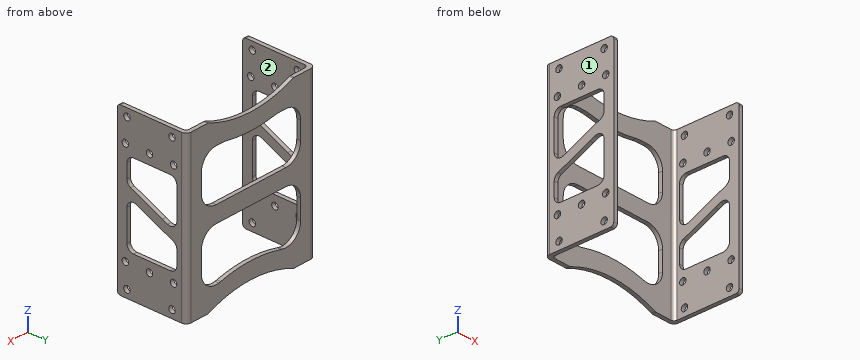
```python
from build123d import *

# Parameters (mm, degrees)
SKETCH_1_W                = 43.5
SKETCH_1_H                = 50
EXTRUDE_1_DEPTH           = 21.5
SKETCH_2_W                = 41.1
SKETCH_2_H                = 22.668209098
CUT_EXTRUDE_1_DEPTH       = 59.078072454
CUT_EXTRUDE_2_DEPTH       = 44.546670366
CUT_EXTRUDE_3_DEPTH       = 44.546670366
HOLE_WIZARD_2_0_2_1_D     = 2
HOLE_WIZARD_2_0_2_1_DEPTH = 1.2
HOLE_WIZARD_2_0_2_2_D     = 2
FILLET_1_R                = 1
FILLET_2_R                = 1.5
FILLET_3_R                = 1
CUT_EXTRUDE_5_DEPTH       = 10
FILLET_4_R                = 10
FILLET_5_R                = 5
CUT_EXTRUDE_6_DEPTH       = 58.037268572
FILLET_6_R                = 2
FILLET_7_R                = 2


with BuildPart() as part:
    # 草图1 → 凸台-拉伸1 (new body)
    with BuildSketch(Plane.XZ.offset(20)):
        with Locations((0, -6)):
            Rectangle(SKETCH_1_W, SKETCH_1_H)
    extrude(amount=-EXTRUDE_1_DEPTH)

    # 草图2 → 切除-拉伸1 (cut, through all)
    with BuildSketch(Plane.XY.offset(19)):
        with Locations((0, -11.034104549)):
            Rectangle(SKETCH_2_W, SKETCH_2_H)
    extrude(amount=-CUT_EXTRUDE_1_DEPTH, mode=Mode.SUBTRACT)

    # 草图3 → 切除-拉伸2 (cut, through all)
    with BuildSketch(Plane(origin=(0, 1.5, 0), x_dir=(-1, 0, 0), z_dir=(0, 1, 0))):
        with BuildLine():
            Line((14.38749457, 19), (-14.38749457, 19))
            ThreePointArc((-14.38749457, 19), (0, 16), (14.38749457, 19))
        make_face()
    extrude(amount=-CUT_EXTRUDE_2_DEPTH, mode=Mode.SUBTRACT)

    # 草图4 → 切除-拉伸3 (cut, through all)
    with BuildSketch(Plane(origin=(0, 1.5, 0), x_dir=(-1, 0, 0), z_dir=(0, 1, 0))):
        with BuildLine():
            Line((-14.38749457, -31), (14.38749457, -31))
            ThreePointArc((14.38749457, -31), (0, -28), (-14.38749457, -31))
        make_face()
    extrude(amount=-CUT_EXTRUDE_3_DEPTH, mode=Mode.SUBTRACT)

    # Ø2.0 (2) 直径孔1
    with Locations(Plane.ZY.offset(-20.55)):
        with Locations((16.6, -3), (16.6, -17), (9.5, -17.5), (9.6, -10), (9.5, -2.5), (-21.5, -2.5), (-28.6, -3), (-28.6, -17), (-21.5, -17.5), (-21.6, -10)):
            Hole(HOLE_WIZARD_2_0_2_1_D / 2, depth=HOLE_WIZARD_2_0_2_1_DEPTH)

    # Ø2.0 (2) 直径孔2 (through all)
    with Locations(Plane(origin=(-20.55, 0, 0), x_dir=(0, 0, -1), z_dir=(1, 0, 0))):
        with Locations((-16.6, -3), (-16.6, -17), (-9.5, -17.5), (-9.6, -10), (-9.5, -2.5), (21.5, -2.5), (28.6, -3), (28.6, -17), (21.5, -17.5), (21.6, -10)):
            Hole(HOLE_WIZARD_2_0_2_2_D / 2)

    # 圆角1
    fillet_1_edges = [part.edges().sort_by_distance(p)[0] for p in [
        (-21.15, -20, 19),
        (21.15, -20, -31),
        (-14.38749457, 0.9, 19),
        (14.38749457, 0.9, 19),
        (-21.15, -20, -31),
        (14.38749457, 0.9, -31),
        (-14.38749457, 0.9, -31),
        (21.15, -20, 19),
    ]]
    fillet(fillet_1_edges, radius=FILLET_1_R)

    # 圆角2
    fillet_2_edges = [part.edges().sort_by_distance(p)[0] for p in [
        (-21.75, 1.5, -6),
        (21.75, 1.5, -6),
    ]]
    fillet(fillet_2_edges, radius=FILLET_2_R)

    # 圆角3
    fillet_3_edges = [part.edges().sort_by_distance(p)[0] for p in [
        (-20.55, 0.3, -6),
        (20.55, 0.3, -6),
    ]]
    fillet(fillet_3_edges, radius=FILLET_3_R)

    # 草图14 → 切除-拉伸5 (cut)
    with BuildSketch(Plane(origin=(0, 1.5, 0), x_dir=(1, 0, 0), z_dir=(0, 1, 0))):
        with BuildLine():
            Line((-11.33348239, 24.597561282), (-16.75, 24.597561282))
            Line((-16.75, 24.597561282), (-16.75, 8.5))
            Line((-16.75, 8.5), (16.75, 8.5))
            Line((16.75, 8.5), (16.75, 24.597561282))
            Line((16.75, 24.597561282), (11.33348239, 24.597561282))
            ThreePointArc((11.33348239, 24.597561282), (0, 23), (-11.33348239, 24.597561282))
        make_face()
        with BuildLine():
            Line((16.75, 3.5), (-16.75, 3.5))
            Line((-16.75, 3.5), (-16.75, -11.921871339))
            Line((-16.75, -11.921871339), (-8.645438281, -11.921871339))
            ThreePointArc((-8.645438281, -11.921871339), (0, -11), (8.645438281, -11.921871339))
            Line((8.645438281, -11.921871339), (16.75, -11.921871339))
            Line((16.75, -11.921871339), (16.75, 3.5))
        make_face()
    extrude(amount=-CUT_EXTRUDE_5_DEPTH, mode=Mode.SUBTRACT)

    # 圆角4
    fillet_4_edges = [part.edges().sort_by_distance(p)[0] for p in [
        (-11.33348239, 0.9, -24.597561282),
        (11.33348239, 0.9, -24.597561282),
        (8.645438281, 0.9, 11.921871339),
        (-8.645438281, 0.9, 11.921871339),
    ]]
    fillet(fillet_4_edges, radius=FILLET_4_R)

    # 圆角5
    fillet_5_edges = [part.edges().sort_by_distance(p)[0] for p in [
        (-16.75, 0.9, 11.921871339),
        (-16.75, 0.9, -3.5),
        (16.75, 0.9, 11.921871339),
        (16.75, 0.9, -3.5),
        (16.75, 0.9, -8.5),
        (16.75, 0.9, -24.597561282),
        (-16.75, 0.9, -8.5),
        (-16.75, 0.9, -24.597561282),
    ]]
    fillet(fillet_5_edges, radius=FILLET_5_R)

    # 草图15 → 切除-拉伸6 (cut, through all)
    with BuildSketch(Plane.ZY.offset(21.75)):
        Polygon((-11, -1.5), (-18.6, -1.5), (-18.6, -17), (-6, -17), (-6, -12.571428571), align=None)
        Polygon((-4, -17), (-6, -12.571428571), (-6, -17), align=None)
        Polygon((6.6, -1.5), (-6, -1.5), (-6, -5.928571429), (-1, -17), (6.6, -17), align=None)
        Polygon((-6, -1.5), (-8, -1.5), (-6, -5.928571429), align=None)
    extrude(amount=-CUT_EXTRUDE_6_DEPTH, mode=Mode.SUBTRACT)

    # 圆角6
    fillet_6_edges = [part.edges().sort_by_distance(p)[0] for p in [
        (-21.15, -1.5, -8),
        (-21.15, -1.5, 6.6),
        (-21.15, -17, 6.6),
        (-21.15, -17, -1),
        (-21.15, -17, -4),
        (-21.15, -17, -18.6),
        (-21.15, -1.5, -18.6),
        (-21.15, -1.5, -11),
    ]]
    fillet(fillet_6_edges, radius=FILLET_6_R)

    # 圆角7
    fillet_7_edges = [part.edges().sort_by_distance(p)[0] for p in [
        (21.15, -1.5, -8),
        (21.15, -1.5, 6.6),
        (21.15, -17, 6.6),
        (21.15, -17, -1),
        (21.15, -17, -4),
        (21.15, -17, -18.6),
        (21.15, -1.5, -18.6),
        (21.15, -1.5, -11),
    ]]
    fillet(fillet_7_edges, radius=FILLET_7_R)


solid = part.part
```
Part model, mm, in its own coordinate system. Face numbers are marked on the shaded views. A direction names the side the tool comes from. Round coordinates to 2 decimals unless told otherwise and drop trailing zeros. Loops run counter-clockwise (first coordinate to the right, second up) from the corner with the lowest first, then second, coordinate; pieces in that order, holes last.
Item 1: Cut at A-A, the plane z = 3.5. Give the cut face in (x, y), then the cut area to 3 significant figures.
Item 2: 3-axis set-ups, long thin cutter, end or side, ignore diameter. For the marked faces 1 and 2: which of +Z, -Z, +X, -X, +Y, -Y reach the whole face in a straight line?
Item 3: Drill centre lines: line 1 (X direction, y = -12.5, z = 15); line 2 (Y direction, x = -20.85, z = 16.6). Where is each one in solid material? Low to high.
Item 4: Cut at C-C, the plane x = 3. Give the cut face in (y, z).
Item 5: Drop flat-ended pins along their axis: P1, Ø2.5, axis at y = -10, z = 9.6, coming from the -X side; P2, Ø0.6, axis at x = -10.5, y = 0.5, coming from the -Z side; P3, Ø0.6, axis at x = -21, z = 2.5, coming from the +Y side. Give the stop position or say it passes through.
Item 6: Cut at B-B, the plane z = 16.6. State how many separate pieces and enclosed holes the cut face has, then the cut area to 3 significant figures.
A:
1. outline: (-21.75, -20) - (-20.55, -20) - (-20.55, -17) - (-21.75, -17) - close; (-21.75, -1.5) - (-20.55, -1.5) - (-20.55, -0.7) arc R1 cw to (-19.55, 0.3) - (-16.75, 0.3) - (-16.75, 1.5) - (-20.25, 1.5) arc R1.5 ccw to (-21.75, 0) - close; (16.75, 0.3) - (19.55, 0.3) arc R1 cw to (20.55, -0.7) - (20.55, -1.5) - (21.75, -1.5) - (21.75, 0) arc R1.5 ccw to (20.25, 1.5) - (16.75, 1.5) - close; (20.55, -20) - (21.75, -20) - (21.75, -17) - (20.55, -17) - close
1. area: 23.0 mm2
2. face 1: +Z, -Z, -X, +Y, -Y
2. face 2: +Z, -Z, -Y
3. line 1: x = -21.75 to -20.55, 20.55 to 21.75
3. line 2: y = -20 to -18, -16 to -4, -2 to 1.37
4. outline: (0.3, -28.13) - (1.5, -28.13) - (1.5, -23.11) - (0.3, -23.11) - close; (0.3, -8.5) - (1.5, -8.5) - (1.5, -3.5) - (0.3, -3.5) - close; (0.3, 11.11) - (1.5, 11.11) - (1.5, 16.13) - (0.3, 16.13) - close
5. P1: stops at x = -21.75
5. P2: stops at z = -29.66
5. P3: stops at y = 1.43
6. separate pieces: 6
6. enclosed holes: 0
6. area: 75.1 mm2
